from build123d import *

# Parameters (mm, degrees)
F0_W     = 30
F0_H     = 50
F1_DEPTH = 20
F3_R     = 1
F4_DEPTH = 18


with BuildPart() as f1:
    # F0 (on Front) → F1 (new body)
    with BuildSketch(Plane.XZ):
        with Locations((15, 25)):
            Rectangle(F0_W, F0_H)
    extrude(amount=F1_DEPTH)

    # F3 (on offset) → F4 (cut)
    with BuildSketch(Plane.XZ.offset(20)):
        with BuildLine():
            Line((2, 48), (2, 2))
            Line((2, 2), (13, 2))
            ThreePointArc((13, 2), (15, 4), (17, 2))
            Line((17, 2), (28, 2))
            Line((28, 2), (28, 48))
            Line((28, 48), (17, 48))
            ThreePointArc((17, 48), (15, 46), (13, 48))
            Line((13, 48), (2, 48))
        make_face()
        with Locations((15, 2)):
            Circle(F3_R)
        with Locations((15, 48)):
            Circle(F3_R)
    extrude(amount=-F4_DEPTH, mode=Mode.SUBTRACT)


solid = f1.part
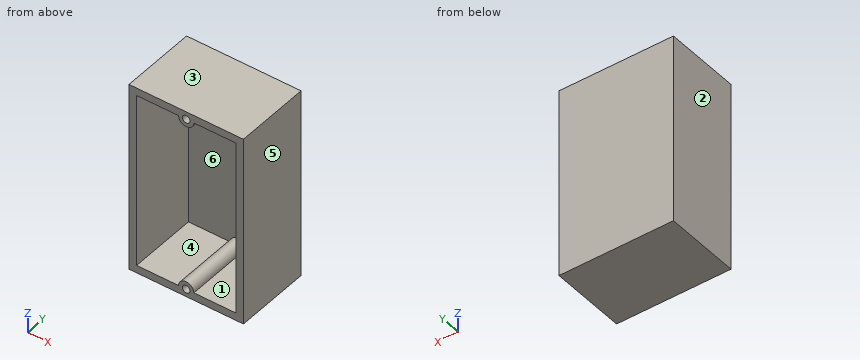
For this review, take the finished solid that the model builds, in its own axes (mm). Face numbers are marked on the shaded views. A direction names the side the tool comes from. Round coordinates to 2 decimals unless told otherwise and drop trailing zeros. Order: outer loops, then holes, each group sorted by start corner. A loop starts at its lowest first (then second) coordinate and runs counter-clockwise, first axis right, second up. Notation, with made-up numbers: (77.25, 19) -> (132.25, 19) arc R17 ccw to (132.25, 47) -> close; hole circle Ø1 at (-4.75, 31). An arc over 180 degrees is marked (long way). Put each result on its own line as item: value.
Q1. Add section B-B on y = -13.5. Write out the cut boundary in (x, z).
Check result:
outline: (0, 0) -> (30, 0) -> (30, 50) -> (0, 50) -> close; hole (2, 2) -> (13, 2) arc R2 cw to (17, 2) -> (28, 2) -> (28, 48) -> (17, 48) arc R2 cw to (13, 48) -> (2, 48) -> close; hole circle Ø2 at (15, 2); hole circle Ø2 at (15, 48)
Q2. For probe 1 along Z at (x, y) = (15, -13); probe 2 along Z at (x, y) = (2.5, -6); probe 3 along X at (y, z) = (-9, 18.5), list the stretches that pass through material, from the lowest coordinate up. Write a range as [from, to].
Check result:
probe 1: [0, 1], [3, 4], [46, 47], [49, 50]
probe 2: [0, 2], [48, 50]
probe 3: [0, 2], [28, 30]
Q3. Add section C-C on x = 18. Write out the cut boundary in (y, z), plus the area to 3 significant figures.
Check result:
outline: (-20, 0) -> (0, 0) -> (0, 50) -> (-20, 50) -> (-20, 48) -> (-2, 48) -> (-2, 2) -> (-20, 2) -> close
area: 172 mm2
Q4. Add section A-A on z = 42.5. Write out the cut boundary in (x, y), plus the area to 3 significant figures.
Check result:
outline: (0, -20) -> (2, -20) -> (2, -2) -> (28, -2) -> (28, -20) -> (30, -20) -> (30, 0) -> (0, 0) -> close
area: 132 mm2
Q5. Insertion check: pin 1 Ø1 at (x, z) = (15, 2) entering from -Y. The pin has a flat end and moves straight along its axis. Give the tip position at first contact, or say it passes through.
Check result:
pin 1: y = -2
Q6. Machinability: for the marked faces 5 and 6, which of the approach directions +Z, -Z, +X, -X, +Y, -Y give a long, thin tool a straight path to every point of the face, cutting with its end or side? Answer none if there is none.
Check result:
face 5: +Z, -Z, +X, +Y, -Y
face 6: -Y
Q7. Mouldability with a two-part tool opening along X and no side actions: class the marked faces 1, 2, 3 and 4 as pulls with the +X half, pulls with the -X half, needs draft (parallel to the pull), parting line crosses it, or undercut.
Check result:
face 1: undercut
face 2: pulls with the -X half
face 3: needs draft
face 4: undercut
